```python
from build123d import *

# Parameters (mm, degrees)
SKETCH2_R          = 8.325
CUT_EXTRUDE2_DEPTH = 10
CHAMFER1_SIZE      = 0.5


with BuildPart() as part:
    # Sketch1 → Revolve1 (revolve)
    with BuildSketch(Plane(origin=(0, 0, 0), x_dir=(1, 0, 0), z_dir=(0, 1, 0))):
        Polygon((1.55, 0), (3, 0), (3, -5), (8.325, -5), (0.325, -13), (0.2, -13), (0.2, -12.5), (1, -10.9), (1, -10), (1, -1), (1.55, -1), align=None)
    revolve(axis=Axis((0, 0, 0), (0, 0, 1)))

    # Sketch2 → Cut-Extrude2 (cut)
    with BuildSketch(Plane(origin=(0, 0, 5), x_dir=(-1, 0, 0), z_dir=(0, 0, -1))):
        Circle(SKETCH2_R)
        Polygon((-4.330127019, 0), (-2.165063509, -3.75), (2.165063509, -3.75), (4.330127019, 0), (2.165063509, 3.75), (-2.165063509, 3.75), align=None, mode=Mode.SUBTRACT)
    extrude(amount=-CUT_EXTRUDE2_DEPTH, mode=Mode.SUBTRACT)

    # Chamfer1
    chamfer1_edges = [part.edges().sort_by_distance(p)[0] for p in [
        (-3, 0, 0),
    ]]
    chamfer(chamfer1_edges, length=CHAMFER1_SIZE)


solid = part.part
```
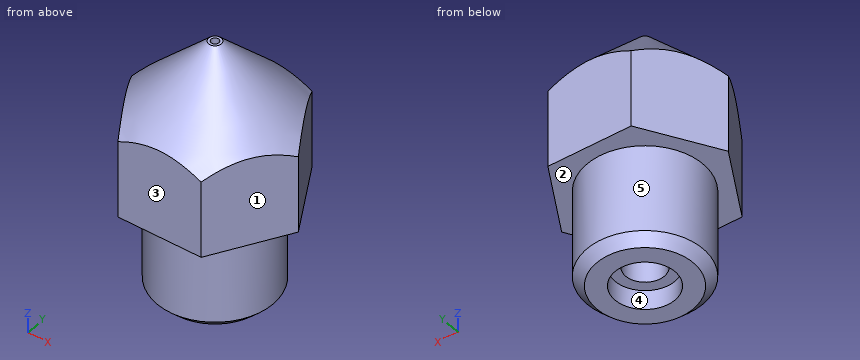
Verification items for the finished model (mm, model axes). Face numbers are marked on the shaded views. A direction names the side the tool comes from. Coordinates: 2 decimals unless noted, no trailing zeros. Loops run counter-clockwise (first coordinate to the right, second up) from the corner with the lowest first, then second, coordinate; pieces in that order, holes last. Notation, with made-up numbers: (44.25, 50) - (48.25, 50) arc R17 cw to (48.25, 74) - close; hole circle Ø10 at (11.5, 88.5). An arc over 180 degrees is marked (long way). Put each result on its own line as item: value.
Item 1: Section check B-B (z = 8.5). Enter the section's corners in (x, y).
Conclusion:
outline: (-4.33, 0) - (-2.17, -3.75) - (2.17, -3.75) - (4.33, 0) - (2.17, 3.75) - (-2.17, 3.75) - close; hole circle Ø2 at (0, 0)
Item 2: Set-up check for the marked faces 1 and 2: record each of +Z, -Z, +X, -X, +Y, -Y from which the full face is reachable in a straight line by a thin tool's end or side.
Conclusion:
face 1: +Z, -Z, +X, -Y
face 2: -Z
Item 3: Section check C-C (z = 2.75). Enter the section's corners in (x, y), then the cut area to 3 significant figures.
Conclusion:
outline: circle Ø6 at (0, 0); hole circle Ø2 at (0, 0)
area: 25.1 mm2
Item 4: Gauge pin test, flat ends, axial feed: pin 1 Ø2.5 at (x, y) = (0, 0) entering from -Z; pin 2 Ø3.5 at (x, y) = (-0.5, 0.5) entering from -Z; pin 3 Ø1 at (x, z) = (-1.5, 10) entering from -Y; pin 4 Ø3 at (y, z) = (2, 8) entering from +X. Record the tip position at first contact, or that the pin passes through.
Conclusion:
pin 1: stops at z = 1
pin 2: stops at z = 0
pin 3: stops at y = -3.55
pin 4: stops at x = 4.04
Item 5: Scan lines: line 1 along Y through (x, z) = (-0.5, 7); line 2 along Y through (x, z) = (-0.5, 4.5); line 3 along X through (y, z) = (-0.5, 6.5). Record each from-to range of solid material in increasing order.
Conclusion:
line 1: y = -3.75 to -0.87, 0.87 to 3.75
line 2: y = -2.96 to -0.87, 0.87 to 2.96
line 3: x = -4.04 to -0.87, 0.87 to 4.04
Item 6: Section check D-D (z = 10.75). Enter the section's corners in (x, y) (3 decimals), then the cut area to 3 significant figures.
Conclusion:
outline: circle Ø5.15 at (0, 0); hole circle Ø2 at (0, 0)
area: 17.7 mm2
Item 7: Section check A-A (x = 0). Enter the section's corners in (y, z) (3 decimals).
Conclusion:
outline: (-3.75, 5) - (-3, 5) - (-3, 0.5) - (-2.5, 0) - (-1.55, 0) - (-1.55, 1) - (-1, 1) - (-1, 10.9) - (-0.2, 12.5) - (-0.2, 13) - (-0.325, 13) - (-3.75, 9.575) - close; (0.2, 12.5) - (1, 10.9) - (1, 1) - (1.55, 1) - (1.55, 0) - (2.5, 0) - (3, 0.5) - (3, 5) - (3.75, 5) - (3.75, 9.575) - (0.325, 13) - (0.2, 13) - close
Item 8: Draft check along Y on the marked faces 3, 4 and 5. Enter one of: pulls with the +Y half, pulls with the -Y half, needs draft (parallel to the pull), parting line crosses it, or undercut.
Conclusion:
face 3: pulls with the -Y half
face 4: undercut
face 5: parting line crosses it
